```python
from build123d import *

# Parameters (mm, degrees)
SKETCH1_R           = 1.5
BOSS_EXTRUDE1_DEPTH = 40
FILLET1_R           = 0.4
SKETCH2_R           = 2.972656176
SKETCH2_R_2         = 1.4
CUT_EXTRUDE1_DEPTH  = 0.15


with BuildPart() as part:
    # Sketch1 → Boss-Extrude1 (new body)
    with BuildSketch(Plane.XY):
        Circle(SKETCH1_R)
    extrude(amount=BOSS_EXTRUDE1_DEPTH)

    # Fillet1
    fillet1_edges = [part.edges().sort_by_distance(p)[0] for p in [
        (-1.5, 0, 0),
        (-1.5, 0, 40),
    ]]
    fillet(fillet1_edges, radius=FILLET1_R)

    # Sketch2 → Cut-Extrude1 (cut)
    with BuildSketch(Plane.XY.offset(25.78)):
        Circle(SKETCH2_R)
        Circle(SKETCH2_R_2, mode=Mode.SUBTRACT)
    extrude(amount=-CUT_EXTRUDE1_DEPTH, mode=Mode.SUBTRACT)


solid = part.part
```
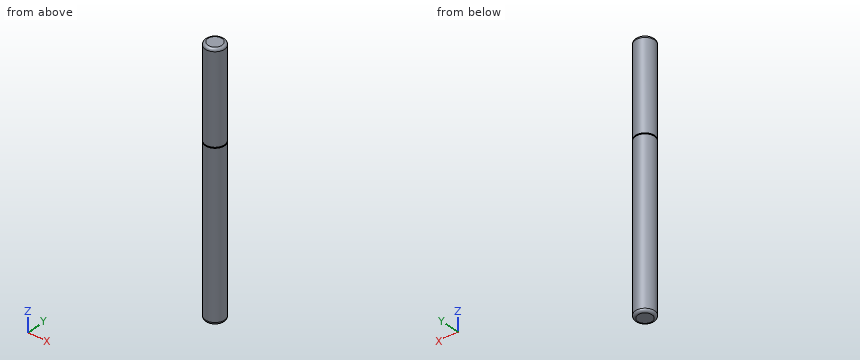
Part model, mm, in its own coordinate system. Round coordinates to 2 decimals unless told otherwise and drop trailing zeros. Order: outer loops, then holes, each group sorted by start corner. A loop starts at its lowest first (then second) coordinate and runs counter-clockwise, first axis right, second up. Notation, with made-up numbers: M 63,42.25 L 90,42.25 A19 cw 90,66.25 Z; hole C 24,22.5 d10. An arc over 180 degrees is marked long. Put each result on its own line as item: value. Start each with the question number.
1. Drop a flat-ended pin along its axis: pin 1 (1.5 mm diameter, centred on x = -0.5, y = -1, fed in from -Z). Give the stop position or say it passes through.
2. Slice it at A-A on z = 13. List the corners of the cut face in (x, y), then the cut area to 3 significant figures.
3. Drill centre lines: probe 1 along Z at (x, y) = (1.1, 0.35); probe 2 along Y at (x, z) = (-0.9, 34); probe 3 along Y at (x, z) = (1.1, 26). Where is each one in solid material? Low to high. Write a range as [from, to].
Findings:
1. pin 1: z = 0
2. outline: C 0,0 d3
2. area: 7.07 mm2
3. probe 1: [0, 40]
3. probe 2: [-1.2, 1.2]
3. probe 3: [-1.02, 1.02]
